Work out the finished part from the listing and answer in its coordinate system (mm). Face numbers are marked on the shaded views. A direction names the side the tool comes from. Round coordinates to 2 decimals unless told otherwise and drop trailing zeros. Order: outer loops, then holes, each group sorted by start corner. A loop starts at its lowest first (then second) coordinate and runs counter-clockwise, first axis right, second up. Notation, with made-up numbers: M 23,38 L 46,38 A29 ccw 46,63 Z; hole C -12.5,52 d8. An arc over 180 degrees is marked long. Return JSON: item names as keys, results as strings.
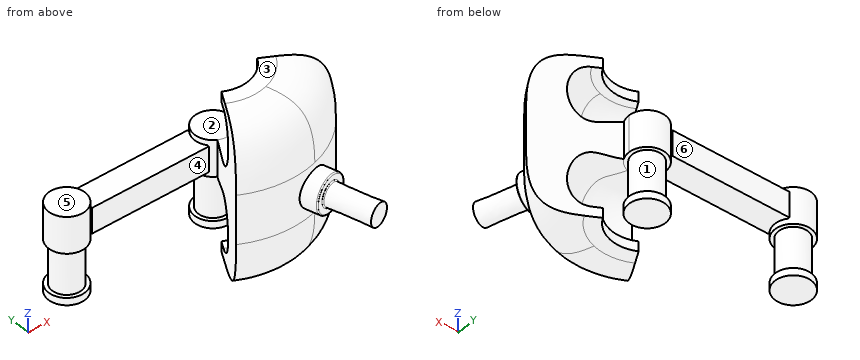
from build123d import *

# Parameters (mm, degrees)
SKETCH10_R          = 25
BOSS_EXTRUDE2_DEPTH = 25
REVOLVE3_ANGLE      = 90
SKETCH19_R          = 25
BOSS_EXTRUDE3_DEPTH = 50
FILLET6_R           = 1.5
SKETCH25_R          = 20
BOSS_EXTRUDE4_DEPTH = 60
BOSS_EXTRUDE5_START = 10
SKETCH26_R          = 25
BOSS_EXTRUDE5_DEPTH = 10
SKETCH27_R          = 20
BOSS_EXTRUDE6_DEPTH = 60
SKETCH28_R          = 25
BOSS_EXTRUDE7_DEPTH = 10


with BuildPart() as part:
    # Sketch3 → Revolve2 (revolve)
    with BuildSketch(Plane(origin=(0, 0, 0), x_dir=(1, 0, 0), z_dir=(0, 1, 0))):
        Polygon((-125, -32.53891123), (-125, 17.46108877), (-100, 17.46108877), (-100, 0), (-100, -15.07782246), (-100, -32.53891123), align=None)
    revolve(axis=Axis((-100, 0, 0), (0, 0, 1)))

    # Sketch6 → Loft2 section 0
    with BuildSketch(Plane(origin=(-80, 0, 0), x_dir=(0, 0, -1), z_dir=(1, 0, 0))):
        with BuildLine():
            Line((9.96108877, -17.5), (-25.03891123, -17.5))
            Line((-25.03891123, -17.5), (-25.03891123, 17.5))
            Line((-25.03891123, 17.5), (9.96108877, 17.5))
            Line((9.96108877, 17.5), (9.96108877, -17.5))
        make_face()
    # Sketch5 → Loft2 section 1
    with BuildSketch(Plane(origin=(80, 0, 0), x_dir=(0, 0, -1), z_dir=(1, 0, 0))):
        with BuildLine():
            Line((9.96108877, -17.5), (-25.03891123, -17.5))
            Line((-25.03891123, -17.5), (-25.03891123, 17.5))
            Line((-25.03891123, 17.5), (9.96108877, 17.5))
            Line((9.96108877, 17.5), (9.96108877, -17.5))
        make_face()
    loft()

    # Sketch10 → Boss-Extrude2 (add, symmetric)
    with BuildSketch(Plane.XY.offset(7.538911233)):
        with Locations((100, 0)):
            Circle(SKETCH10_R)
    extrude(amount=BOSS_EXTRUDE2_DEPTH, both=True)

    # Sketch13 → Revolve3 (revolve, symmetric)
    with BuildSketch(Plane(origin=(92.307490084, 26.647256571, 0), x_dir=(0, 0, -1), z_dir=(0.9607678704250572, 0.27735374372613175, 0))) as revolve3_sk:
        with BuildLine():
            Line((-41.003397863, -157.420055221), (25.925575398, -157.420055221))
            add(Edge.make_bspline(
                [(100.918479625, -95.235374373), (100.918479625, -103.819187393), (98.943583911, -138.760414592), (77.566461401, -157.420055221), (25.925575398, -157.420055221)],
                knots=[0, 0, 0, 0, 0.2175197, 1, 1, 1, 1], degree=3))
            Line((100.918479625, -95.235374373), (100.918479625, -75.235374373))
            Line((100.918479625, -75.235374373), (87.386654253, -75.235374373))
            Line((87.386654253, -75.235374373), (87.386654253, -87.235374373))
            add(Edge.make_bspline(
                [(17.461088767, -52.735374373), (17.461088767, -66.865072707), (2.602893469, -96.99328028), (54.696104455, -123.255260317), (87.386654253, -103.260979897), (87.386654253, -87.235374373)],
                knots=[0, 0, 0, 0, 0.304904739, 0.682398106, 1, 1, 1, 1], degree=3))
            Line((17.461088767, -52.735374373), (-32.538911233, -52.735374373))
            add(Edge.make_bspline(
                [(-32.538911233, -52.735374373), (-32.538911233, -66.865072707), (-17.680715934, -96.99328028), (-69.77392692, -123.255260317), (-102.464476718, -103.260979897), (-102.464476718, -87.235374373)],
                knots=[0, 0, 0, 0, 0.304904739, 0.682398106, 1, 1, 1, 1], degree=3))
            Line((-102.464476718, -87.235374373), (-102.464476718, -75.235374373))
            Line((-102.464476718, -75.235374373), (-115.99630209, -75.235374373))
            Line((-115.99630209, -75.235374373), (-115.99630209, -95.235374373))
            add(Edge.make_bspline(
                [(-115.99630209, -95.235374373), (-115.99630209, -103.819187393), (-114.021406376, -138.760414592), (-92.644283866, -157.420055221), (-41.003397863, -157.420055221)],
                knots=[0, 0, 0, 0, 0.2175197, 1, 1, 1, 1], degree=3))
        make_face()
    revolve(axis=Axis((100, 0, 32.538911233), (0, 0, -1)), revolution_arc=REVOLVE3_ANGLE / 2)
    revolve(revolve3_sk.sketch, axis=Axis((100, 0, 32.538911233), (0, 0, 1)), revolution_arc=REVOLVE3_ANGLE / 2)

    # Sketch19 → Boss-Extrude3 (add)
    with BuildSketch(Plane(origin=(35.427884289, -122.724043613, 0), x_dir=(-0.9607678704226367, -0.27735374373451605, 0), z_dir=(0.27735374373451605, -0.9607678704226368, 0))):
        with Locations((-96.076787042, -7.538911233)):
            Circle(SKETCH19_R)
    extrude(amount=BOSS_EXTRUDE3_DEPTH)

    # Loft4: read off the stored shape, not the designer's step
    # Loft4: loft between two sections, ruled curve by curve
    loft4_from = [
        Edge.make_bspline([(127.882970281, -148.075886157, 12.129325865), (119.062324499, -150.622223525, -16.431352943), (146.502507055, -142.700812334, -25.612182209), (155.323152838, -140.154474966, 2.9484966), (164.14379862, -137.608137599, 31.509175408), (136.703616063, -145.52954879, 40.690004674), (127.882970281, -148.075886157, 12.129325865)], [0, 0, 0, 0, 0.5, 0.5, 0.5, 1, 1, 1, 1], 3, [1, 0.333333333, 0.333333333, 1, 0.333333333, 0.333333333, 1]),
    ]
    loft4_to = [
        Edge.make_bspline([(148.940358563, -205.753913799, 18.677671161), (127.536833252, -211.932667332, -1.41491725), (146.841146631, -206.359912715, -23.692437107), (168.244671942, -200.181159182, -3.599848696), (189.648197253, -194.002405649, 16.492739715), (170.343883874, -199.575160266, 38.770259572), (148.940358563, -205.753913799, 18.677671161)], [0, 0, 0, 0, 0.5, 0.5, 0.5, 1, 1, 1, 1], 3, [1, 0.333333333, 0.333333333, 1, 0.333333333, 0.333333333, 1]),
    ]
    loft4 = Solid(Shell([*[Face.make_surface_from_curves(loft4_from[k], loft4_to[k]) for k in range(1)], Face(Wire(loft4_from)), Face(Wire(loft4_to))]))
    add(loft4)

    # Fillet6
    fillet6_edges = [part.edges().sort_by_distance(p)[0] for p in [
        (165.62225832, -137.181336969, 7.538911233),
        (155.323152838, -140.154474966, 2.9484966),
    ]]
    fillet(fillet6_edges, radius=FILLET6_R)

    # Sketch25 → Boss-Extrude4 (add)
    with BuildSketch(Plane(origin=(0, 0, -17.46108877), x_dir=(-1, 0, 0), z_dir=(0, 0, -1))):
        with Locations((100, 0)):
            Circle(SKETCH25_R)
    extrude(amount=BOSS_EXTRUDE4_DEPTH)

    # Sketch26 → Boss-Extrude5 (add)
    with BuildSketch(Plane(origin=(0, 0, -77.46108877), x_dir=(-1, 0, 0), z_dir=(0, 0, -1)).offset(BOSS_EXTRUDE5_START)):
        with Locations((100, 0)):
            Circle(SKETCH26_R)
    extrude(amount=-BOSS_EXTRUDE5_DEPTH)

    # Sketch27 → Boss-Extrude6 (add)
    with BuildSketch(Plane(origin=(0, 0, -17.461088767), x_dir=(-1, 0, 0), z_dir=(0, 0, -1))):
        with Locations(Location((-100, 0, 0), (0, 0, 180))):
            Circle(SKETCH27_R)
    extrude(amount=BOSS_EXTRUDE6_DEPTH)

    # Sketch28 → Boss-Extrude7 (add)
    with BuildSketch(Plane(origin=(0, 0, -77.461088767), x_dir=(-1, 0, 0), z_dir=(0, 0, -1))):
        with Locations((-100, 0)):
            Circle(SKETCH28_R)
    extrude(amount=BOSS_EXTRUDE7_DEPTH)


solid = part.part
Item 1: Each of these flat-tipped pins is pushed along its axis until it touches: pin 1 (10.5 mm diameter, centred on x = -18.5, y = -3, fed in from -Z); pin 2 (15 mm diameter, centred on x = -99.5, y = 11, fed in from -Z); pin 3 (17.5 mm diameter, centred on x = -3, y = -7.5, fed in from +Z). Where does it stop, or does it pass through?
Output:
{"pin 1": "stops at z = -9.96", "pin 2": "stops at z = -87.46", "pin 3": "stops at z = 25.04"}
Item 2: Find section C-C (x = -40). Determine the outline of the cut face in (y, z).
Output:
{"outline": "M -17.5,-9.96 L 17.5,-9.96 L 17.5,25.04 L -17.5,25.04 Z"}
Item 3: Find section A-A (x = -100). Determine the outline of the cut face in (y, z), plus the area to 3 significant figures.
Output:
{"outline": "M -25,-87.46 L 25,-87.46 L 25,-77.46 L 20,-77.46 L 20,-17.46 L 25,-17.46 L 25,32.54 L -25,32.54 L -25,-17.46 L -20,-17.46 L -20,-77.46 L -25,-77.46 Z", "area": "5,400 mm^2"}
Item 4: Which of the six approach directions +Z, -Z, +X, -X, +Y, -Y give full straight-line access (tool end or side, diameter ignored) to the marked faces 1, 2 and 3?
Output:
{"face 1": "none", "face 2": "+Z, +X, -X, +Y", "face 3": "+Z, +X, -X, +Y, -Y"}
Item 5: Find section B-B (z = -62). State how many separate pieces and enclosed holes the cut face has, plus the area to 3 significant figures.
Output:
{"separate pieces": "3", "enclosed holes": "0", "area": "9,340 mm^2"}
Item 6: Consider line 1 along Z through (x, y) = (16, -3); line 2 along Y through (x, z) = (104, -65); line 3 along Z through (x, y) = (119, 2). Determine where each line is inside the solid, lowest interval first. Write a range as [from, to].
Output:
{"line 1": "z = [-9.96, 25.04]", "line 2": "y = [-125.43, -84.35], [-19.6, 19.6]", "line 3": "z = [-87.46, 32.54]"}
Item 7: The mould has two halves that part along Y. Classify the marked faces 4, 5 and 6: pulls with the +Y half, pulls with the -Y half, needs draft (parallel to the pull), parting line crosses it, or undercut.
Output:
{"face 4": "undercut", "face 5": "needs draft", "face 6": "pulls with the +Y half"}
